Geometry: see drawing. Coordinates: mm, zero at the bounding-box minimum. A direction names the side the tool comes from. Coordinates: 2 decimals unless noted, no trailing zeros. Order: outer loops, then holes, each group sorted by start corner. A loop starts at its lowest first (then second) coordinate and runs counter-clockwise, first axis right, second up. Notation, with made-up numbers: M -31.5,80 L 8.5,80 A31 ccw 8.5,104 Z; hole C 4,-19.75 d6. An arc over 180 degrees is marked long. Answer in a Markdown table with one row per item.
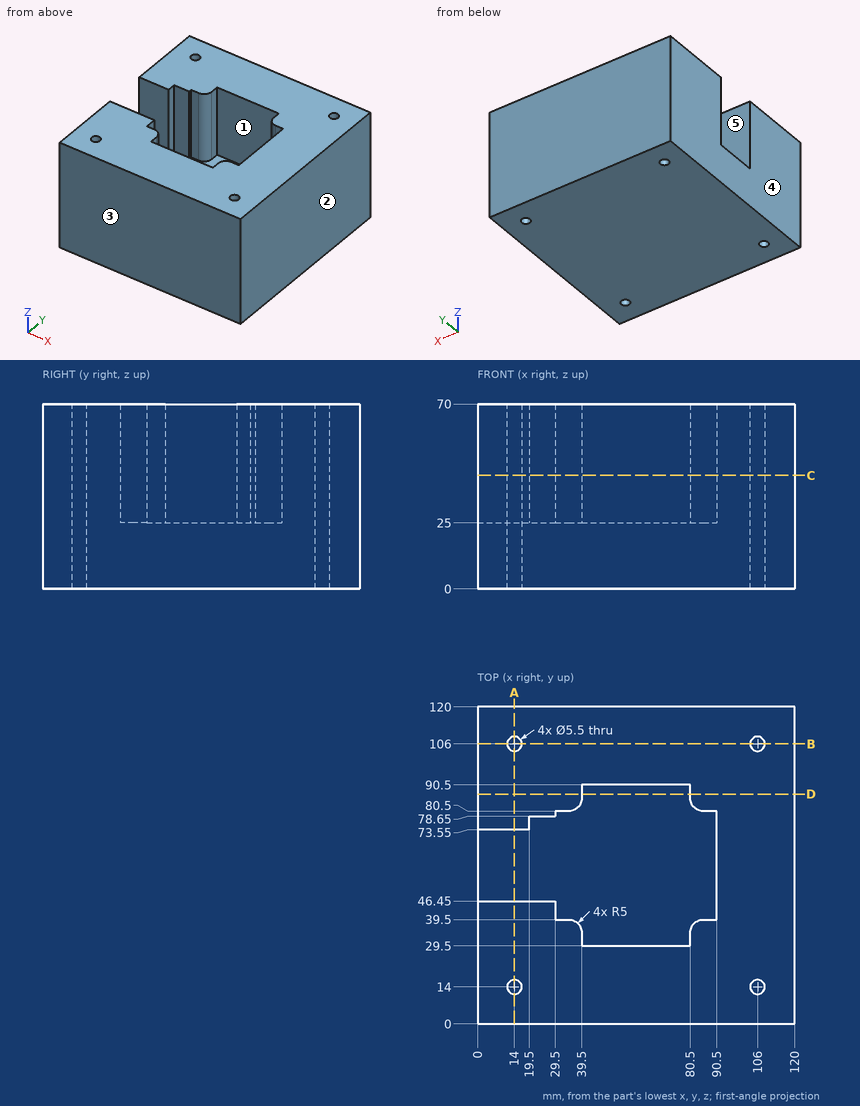
1) Mould query, pull axis Y, two halves, no side actions, for the marked faces 1, 2 and 3. Classes: +Y half, -Y half, draft (parallel to the pull), parting line (faces both ways), or undercut.
Resolved:
| item | result |
|---|---|
| face 1 | undercut |
| face 2 | draft |
| face 3 | -Y half |
2) Cut plane B-B, the plane y = 106. Output: boundary loops of the cut face in (x, z), and give its area (3 significant figures).
Resolved:
| item | result |
|---|---|
| outline | M 0,0 L 11.25,0 L 11.25,70 L 0,70 Z; M 16.75,0 L 103.25,0 L 103.25,70 L 16.75,70 Z; M 108.75,0 L 120,0 L 120,70 L 108.75,70 Z |
| area | 7,630 mm2 |
3) Cut plane D-D, the plane y = 87. Output: boundary loops of the cut face in (x, z).
Resolved:
| item | result |
|---|---|
| outline | M 0,0 L 120,0 L 120,70 L 80.5,70 L 80.5,25 L 39.5,25 L 39.5,70 L 0,70 Z |
4) Reachability of the marked faces 4 and 5 from +Z, -Z, +X, -X, +Y, -Y: full face, straight path, thin tool, end or side. Return the list, or none.
Resolved:
| item | result |
|---|---|
| face 4 | +Z, -Z, -X, +Y, -Y |
| face 5 | +Z, -X |
5) Cut plane C-C, the plane z = 43. State how many separate pieces and enclosed holes the cut face has, and give its area (3 significant figures).
Resolved:
| item | result |
|---|---|
| separate pieces | 1 |
| enclosed holes | 4 |
| area | 10,100 mm2 |
6) Material intervals for probe 1 along X at (y, z) = (106, 53.5); probe 2 along X at (y, z) = (33.5, 35), sorted ascending.
Resolved:
| item | result |
|---|---|
| probe 1 | x = 0 to 11.25, 16.75 to 103.25, 108.75 to 120 |
| probe 2 | x = 0 to 39.5, 80.5 to 120 |
7) Cut plane A-A, the plane x = 14. Output: boundary loops of the cut face in (y, z).
Resolved:
| item | result |
|---|---|
| outline | M 0,0 L 11.25,0 L 11.25,70 L 0,70 Z; M 16.75,0 L 103.25,0 L 103.25,70 L 73.55,70 L 73.55,25 L 46.45,25 L 46.45,70 L 16.75,70 Z; M 108.75,0 L 120,0 L 120,70 L 108.75,70 Z |
